Could you check a few things on this model? Use its own coordinates, in mm. A direction names the side the tool comes from. Give positions to 0.01 mm unless a question says otherwise; leave off trailing zeros. Order: outer loops, then holes, each group sorted by start corner. A loop starts at its lowest first (then second) coordinate and runs counter-clockwise, first axis right, second up.
(1) Imagine slicing it at A-A, the plane z = 0. Write out the boundary of the cut face in (x, y).
(2) Imagine slicing it at B-B, the plane y = 18.5. Write out the boundary of the cut face in (x, z), then the cut area to 3 significant figures.
(3) Imagine slicing it at C-C, the plane y = 10.5. Write out the boundary of the cut face in (x, z).
(4) Will these pins go through, and if not, where does the flat tip stop? pin 1 (1 mm diameter, centred on y = 2.5, z = -14, fed in from -X); pin 2 (1.5 mm diameter, centred on y = 14.5, z = 12.5, fed in from -X); pin 3 (1.1 mm diameter, centred on y = 8.5, z = 15, fed in from -X).
(5) Imagine slicing it at D-D, the plane z = -13.5. State how many separate pieces and enclosed holes the cut face has, then the cut area to 3 significant figures.
(6) On a 3-axis mill with a long thin cutter (end or side, diameter ignored), from which of +Z, -Z, +X, -X, +Y, -Y can I reach the whole of each face in a straight line? I mean faces 1 (the flat face through (24.4, 7.58, 17.84)), 2 (the flat face through (17, 3, -31)), 3 (the flat face through (-26, 9.2, 15)), 4 (the cylindrical face through (0, 7.6, -24.5)), 5 (the cylindrical face through (23.91, 8.06, -11.83)). Say none if no direction works.
(7) If I drill on probe 1 along Y at (x, z) = (25, 12); probe 2 along Z at (x, y) = (-22.5, 5.5); probe 3 along X at (y, z) = (8.5, -13.5), over which ranges is the centre line in solid material (lowest first)?
(8) If we mould it in two halves opening along Y, with no side actions, what happens to faces 6 (the flat face through (22, 20, 12)), 7 (the flat face through (-3.25, 8, -30)), 8 (the cylindrical face through (24.5, 5, 12.5))? For each: released by +Y, released by -Y, zero draft, split by the parting line, or undercut.
from build123d import *

# Parameters (mm, degrees)
SKETCH1_R                       = 37.5
BOSS_EXTRUDE1_DEPTH             = 3
SKETCH1_3_R                     = 35
BOSS_EXTRUDE2_DEPTH             = 12
SKETCH4_R                       = 15.5
CUT_EXTRUDE1_DEPTH              = 15
BOSS_EXTRUDE3_DEPTH             = 3
SKETCH18_R                      = 5
BOSS_EXTRUDE4_DEPTH             = 5
CHAMFER1_SIZE                   = 9
F_3_0MM_DOWEL_HOLE1_D           = 3
F_3_0MM_DOWEL_HOLE1_CSINK_D     = 3.05
F_3_0MM_DOWEL_HOLE1_CSINK_ANGLE = 90
SKETCH27_R                      = 1.75
CUT_EXTRUDE2_DEPTH              = 55.373706881
CUT_EXTRUDE3_START              = -6
SKETCH28_R                      = 1.5
CUT_EXTRUDE3_DEPTH              = 3.2
CIRPATTERN1_COUNT               = 3
SKETCH29_R                      = 32.5
CUT_EXTRUDE4_DEPTH              = 4
CHAMFER2_SIZE                   = 2


with BuildPart() as part:
    # Sketch1 → Boss-Extrude1 (new body)
    with BuildSketch(Plane(origin=(0, 0, 0), x_dir=(1, 0, 0), z_dir=(0, 1, 0))):
        with Locations(Location((0, 0, 0), (0, 0, 270))):
            Circle(SKETCH1_R)
    extrude(amount=BOSS_EXTRUDE1_DEPTH)

    # Sketch1<3> → Boss-Extrude2 (add)
    with BuildSketch(Plane(origin=(0, 0, 0), x_dir=(1, 0, 0), z_dir=(0, 1, 0))):
        with Locations(Location((0, 0, 0), (0, 0, 270))):
            Circle(SKETCH1_3_R)
    extrude(amount=BOSS_EXTRUDE2_DEPTH)

    # Sketch4 → Cut-Extrude1 (cut)
    with BuildSketch(Plane(origin=(0, 12, 0), x_dir=(1, 0, 0), z_dir=(0, 1, 0))):
        with Locations(Location((0, 0, 0), (0, 0, 270))):
            Circle(SKETCH4_R)
    extrude(amount=-CUT_EXTRUDE1_DEPTH, mode=Mode.SUBTRACT)

    # Sketch5 → Boss-Extrude3 (add)
    with BuildSketch(Plane(origin=(0, 12, 0), x_dir=(1, 0, 0), z_dir=(0, 1, 0))):
        with BuildLine():
            ThreePointArc((5.813043417, 34.513888889), (0, 35), (-5.813043417, 34.513888889))
            ThreePointArc((-5.813043417, 34.513888889), (0, 17.5), (5.813043417, 34.513888889))
        make_face()
        with BuildLine():
            ThreePointArc((-26.900782734, -22.390799188), (-15.223614965, -8.789358198), (-32.841392275, -12.101361636))
            ThreePointArc((-32.841392275, -12.101361636), (-30.310889132, -17.5), (-26.900782734, -22.390799188))
        make_face()
        with BuildLine():
            ThreePointArc((26.885233446, -22.409467253), (30.266672739, -17.576362574), (32.7884636, -12.244045686))
            ThreePointArc((32.7884636, -12.244045686), (15.167446159, -8.807989412), (26.885233446, -22.409467253))
        make_face()
    extrude(amount=BOSS_EXTRUDE3_DEPTH)

    # Sketch18 → Boss-Extrude4 (add)
    with BuildSketch(Plane(origin=(0, 15, 0), x_dir=(1, 0, 0), z_dir=(0, 1, 0))):
        with Locations(Location((0, 27, 0), (0, 0, 270))):
            Circle(SKETCH18_R)
        with Locations(Location((23.382685902, -13.5, 0), (0, 0, 270))):
            Circle(SKETCH18_R)
        with Locations(Location((-23.382685902, -13.5, 0), (0, 0, 270))):
            Circle(SKETCH18_R)
    extrude(amount=BOSS_EXTRUDE4_DEPTH)

    # Chamfer1
    chamfer1_edges = [part.edges().sort_by_distance(p)[0] for p in [
        (0, 0, -15.5),
    ]]
    chamfer(chamfer1_edges, length=CHAMFER1_SIZE)

    # Ø3.0mm Dowel Hole1 (through all)
    with Locations(Plane(origin=(0, 20, 0), x_dir=(1, 0, 0), z_dir=(0, 1, 0))):
        with Locations((0, 27), (-23.382685902, -13.5), (23.382685902, -13.5)):
            CounterSinkHole(F_3_0MM_DOWEL_HOLE1_D / 2, F_3_0MM_DOWEL_HOLE1_CSINK_D / 2, counter_sink_angle=F_3_0MM_DOWEL_HOLE1_CSINK_ANGLE)

    # Sketch27 → Cut-Extrude2 (cut, through all)
    with BuildSketch(Plane(origin=(0, 12, 0), x_dir=(1, 0, 0), z_dir=(0, 1, 0))):
        with Locations(Location((23.382685902, 13.5, 0), (0, 0, 270))):
            Circle(SKETCH27_R)
        with Locations(Location((0, -27, 0), (0, 0, 270))):
            Circle(SKETCH27_R)
        with Locations(Location((-23.382685902, 13.5, 0), (0, 0, 270))):
            Circle(SKETCH27_R)
    extrude(amount=-CUT_EXTRUDE2_DEPTH, mode=Mode.SUBTRACT)

    # Sketch28 → Cut-Extrude3 (cut)
    # profile 1 of 2: a face of its own
    with BuildSketch(Plane.XZ.offset(CUT_EXTRUDE3_START)):
        with BuildLine():
            Line((3.25, -37.358901215), (3.25, -28.876388375))
            Line((3.25, -28.876388375), (0, -30.75277675))
            Line((0, -30.75277675), (-3.25, -28.876388375))
            Line((-3.25, -28.876388375), (-3.25, -37.358901215))
            ThreePointArc((-3.25, -37.358901215), (0, -37.5), (3.25, -37.358901215))
        make_face()
    # profile 2 of 2: a face of its own
    with BuildSketch(Plane.XZ.offset(CUT_EXTRUDE3_START)):
        with BuildLine():
            Line((3.25, -28.876388375), (3.25, -25.123611625))
            Line((3.25, -25.123611625), (2.024716505, -24.41619387))
            ThreePointArc((2.024716505, -24.41619387), (0, -24.5), (-2.024716505, -24.41619387))
            Line((-2.024716505, -24.41619387), (-3.25, -25.123611625))
            Line((-3.25, -25.123611625), (-3.25, -28.876388375))
            Line((-3.25, -28.876388375), (0, -30.75277675))
            Line((0, -30.75277675), (3.25, -28.876388375))
        make_face()
        with Locations(Location((0, -27, 0), (0, 0, 90))):
            Circle(SKETCH28_R, mode=Mode.SUBTRACT)
    cut_extrude3 = extrude(amount=-CUT_EXTRUDE3_DEPTH, mode=Mode.SUBTRACT)

    # CirPattern1: Cut-Extrude3 ×3 about axis
    cirpattern1_axis = Axis((0, 0, 0), (0, 1, 0))
    for i in range(1, CIRPATTERN1_COUNT):
        add(cut_extrude3.rotate(cirpattern1_axis, i * 360 / CIRPATTERN1_COUNT), mode=Mode.SUBTRACT)

    # Sketch29 → Cut-Extrude4 (cut)
    with BuildSketch(Plane.XZ):
        with Locations(Location((0, 0, 0), (0, 0, 270))):
            Circle(SKETCH29_R)
    extrude(amount=-CUT_EXTRUDE4_DEPTH, mode=Mode.SUBTRACT)

    # Chamfer2
    chamfer2_edges = [part.edges().sort_by_distance(p)[0] for p in [
        (0, 4, 32.5),
    ]]
    chamfer(chamfer2_edges, length=CHAMFER2_SIZE)


solid = part.part
Answer block:
1. outline: (-37.5, 0) - (-32.5, 0) - (-32.5, 2) - (-30.5, 4) - (-20.5, 4) - (-15.5, 9) - (-15.5, 12) - (-35, 12) - (-35, 3) - (-37.5, 3) - close; (15.5, 9) - (20.5, 4) - (30.5, 4) - (32.5, 2) - (32.5, 0) - (37.5, 0) - (37.5, 3) - (35, 3) - (35, 12) - (15.5, 12) - close
2. outline: circle Ø10 at (-23.38, 13.5); circle Ø10 at (0, -27); circle Ø10 at (23.38, 13.5); hole circle Ø3 at (-23.38, 13.5); hole circle Ø3 at (0, -27); hole circle Ø3 at (23.38, 13.5)
2. area: 214 mm2
3. outline: circle Ø70 at (0, 0); hole circle Ø3.5 at (-23.38, -13.5); hole circle Ø3 at (-23.38, 13.5); hole circle Ø31 at (0, 0); hole circle Ø3.5 at (0, 27); hole circle Ø3 at (0, -27); hole circle Ø3.5 at (23.38, -13.5); hole circle Ø3 at (23.38, 13.5)
4. pin 1: stops at x = -34.99
4. pin 2: stops at x = -32.84
4. pin 3: stops at x = -31.88
5. separate pieces: 4
5. enclosed holes: 0
5. area: 340 mm2
6. face 1: +X
6. face 2: +Y
6. face 3: none
6. face 4: -Z
6. face 5: +Y, -Y
7. probe 1: y = 4 to 6, 9.2 to 20
7. probe 2: z = -26.81 to -15.01, -11.99 to 12.29, 14.71 to 26.81
7. probe 3: x = -32.29 to -25.13, -21.63 to -8.59, 8.59 to 21.63, 25.13 to 32.29
8. face 6: released by +Y
8. face 7: undercut
8. face 8: zero draft
